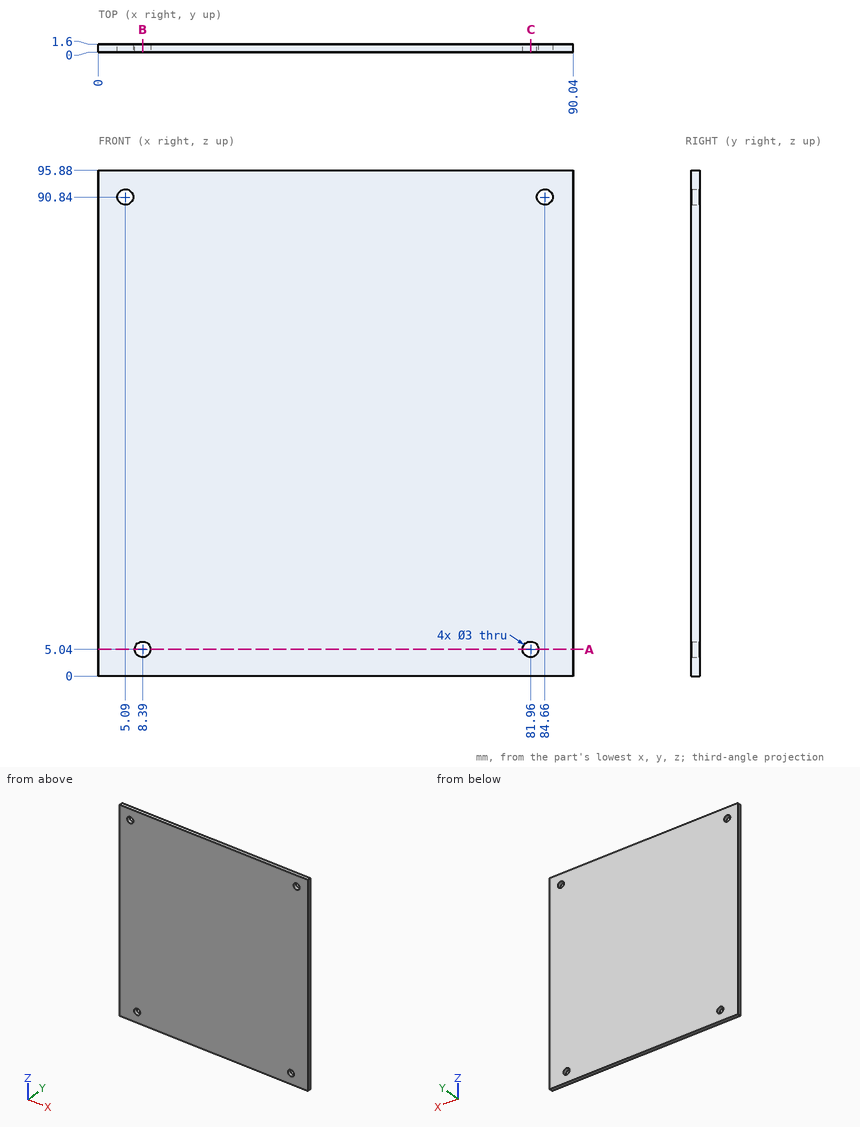
The drawing under review shows one solid part. Ordinate dimensions are in mm from its lowest x, y, z. Round coordinates to 2 decimals unless told otherwise and drop trailing zeros. Loops run counter-clockwise (first coordinate to the right, second up) from the corner with the lowest first, then second, coordinate; pieces in that order, holes last. Notation, with made-up numbers: (-7, -24.5) -> (49, -24.5) arc R24 cw to (49, -10.5) -> close; hole circle Ø9 at (6.25, 59). An arc over 180 degrees is marked (long way). Answer in a Markdown table with one row per item.
1) Wall thickness on line 1 along X through (y, z) = (1.2, 90.84); line 2 along Z through (x, y) = (81.96, 0.5); line 3 along Z through (x, y) = (81, 0.85): over which ranges is each line inside the solid? List them lowest first.
Taken from the geometry:
| item | result |
|---|---|
| line 1 | x = 0 to 3.59, 6.59 to 83.16, 86.16 to 90.04 |
| line 2 | z = 0 to 3.54, 6.54 to 95.88 |
| line 3 | z = 0 to 3.89, 6.19 to 95.88 |
2) Consider section A-A, the plane z = 5.04. Write out the cut boundary in (x, y).
Taken from the geometry:
| item | result |
|---|---|
| outline | (0, 0) -> (6.89, 0) -> (6.89, 1.6) -> (0, 1.6) -> close; (9.89, 0) -> (80.46, 0) -> (80.46, 1.6) -> (9.89, 1.6) -> close; (83.46, 0) -> (90.04, 0) -> (90.04, 1.6) -> (83.46, 1.6) -> close |
3) Consider section B-B, the plane x = 8.39. Write out the cut boundary in (y, z), plus the area to 3 significant figures.
Taken from the geometry:
| item | result |
|---|---|
| outline | (0, 0) -> (1.6, 0) -> (1.6, 3.54) -> (0, 3.54) -> close; (0, 6.54) -> (1.6, 6.54) -> (1.6, 95.88) -> (0, 95.88) -> close |
| area | 149 mm² |
